Verification items for the finished model (mm, model axes). Face numbers are marked on the shaded views. Coordinates: 2 decimals unless noted, no trailing zeros. Order: outer loops, then holes, each group sorted by start corner. A loop starts at its lowest first (then second) coordinate and runs counter-clockwise, first axis right, second up. Notation, with made-up numbers: M 48,-15 L 103,-15 A18 cw 103,6 Z; hole C -22.75,57.25 d7. An arc over 180 degrees is marked long. Return JSON: item names as keys, results as strings.
```python
from build123d import *

# Parameters (mm, degrees)
SKETCH1_R                  = 63
SKETCH1_R_2                = 58
BOSS_EXTRUDE1_DEPTH        = 29.4
SKETCH2_R                  = 60.5
SKETCH2_R_2                = 58
CUT_EXTRUDE1_DEPTH         = 2
BOSS_EXTRUDE2_REACH        = 115.821
BOSS_EXTRUDE2_START_RADIUS = 63
BOSS_EXTRUDE2_END_RADIUS   = 63
SKETCH3_W                  = 60
SKETCH3_H                  = 29.4
SKETCH5_W                  = 29.4
SKETCH5_H                  = 24.463774017
CUT_EXTRUDE2_DEPTH         = 60
BOSS_EXTRUDE3_DEPTH        = 60
SKETCH7_W                  = 60
SKETCH7_H                  = 41.577878734
BOSS_EXTRUDE4_DEPTH        = 50
CUT_EXTRUDE3_REACH         = 173.878
SKETCH9_W                  = 60
SKETCH9_H                  = 50
BOSS_EXTRUDE5_DEPTH        = 26.14
SKETCH10_W                 = 60
SKETCH10_H                 = 26.14
BOSS_EXTRUDE6_DEPTH        = 30
SKETCH11_R                 = 58
CUT_EXTRUDE4_DEPTH         = 168.932327916
SKETCH14_W                 = 60
SKETCH14_H                 = 55.370879129
CUT_EXTRUDE5_DEPTH         = 14.7
CUT_EXTRUDE6_REACH         = 171.856
BOSS_EXTRUDE7_DEPTH        = 60
SKETCH17_R                 = 58
CUT_EXTRUDE7_DEPTH         = 155.195379415
SKETCH18_W                 = 60
SKETCH18_H                 = 15
CUT_EXTRUDE8_DEPTH         = 50
SKETCH19_R                 = 2
CUT_EXTRUDE9_DEPTH         = 15
SKETCH20_W                 = 60
SKETCH20_H                 = 20
CUT_EXTRUDE10_DEPTH        = 140.943357594


with BuildPart() as part:
    # Sketch1 → Boss-Extrude1 (new body)
    with BuildSketch(Plane.XY):
        Circle(SKETCH1_R)
        Circle(SKETCH1_R_2, mode=Mode.SUBTRACT)
    extrude(amount=BOSS_EXTRUDE1_DEPTH)

    # Sketch2 → Cut-Extrude1 (cut)
    with BuildSketch(Plane.XY.offset(29.4)):
        Circle(SKETCH2_R)
        Circle(SKETCH2_R_2, mode=Mode.SUBTRACT)
    extrude(amount=-CUT_EXTRUDE1_DEPTH, mode=Mode.SUBTRACT)

    # Boss-Extrude2: from a cylinder face, 115.821 long prism both ways, kept between that surface and its translate by the depth
    boss_extrude2_start = Plane(origin=(0, 0, 14.7), z_dir=(0, 0, -1)) * Cylinder(BOSS_EXTRUDE2_START_RADIUS, 358.642, mode=Mode.PRIVATE)
    boss_extrude2_end = Plane(origin=(0, 20, 14.7), z_dir=(0, 0, -1)) * Cylinder(BOSS_EXTRUDE2_END_RADIUS, 358.642, mode=Mode.PRIVATE)
    # Sketch3 → Boss-Extrude2 (add, from a surface)
    with BuildSketch(Plane(origin=(0, 0, 0), x_dir=(1, 0, 0), z_dir=(0, 1, 0)), mode=Mode.PRIVATE) as boss_extrude2_sk1:
        with Locations((0, -14.7)):
            Rectangle(SKETCH3_W, SKETCH3_H)
    boss_extrude2_tool1 = extrude(boss_extrude2_sk1.sketch, amount=BOSS_EXTRUDE2_REACH, both=True, mode=Mode.PRIVATE)
    add(((boss_extrude2_tool1 - boss_extrude2_start) & boss_extrude2_end).solids().sort_by_distance((0, 65.398556, 14.7))[0])

    # Sketch5 → Cut-Extrude2 (cut)
    with BuildSketch(Plane.ZY.offset(30)):
        with Locations((14.7, 87.630442947)):
            Rectangle(SKETCH5_W, SKETCH5_H)
    extrude(amount=-CUT_EXTRUDE2_DEPTH, mode=Mode.SUBTRACT)

    # Sketch6 → Boss-Extrude3 (add)
    with BuildSketch(Plane.ZY.offset(30)):
        Polygon((0, 75.398555938), (29.4, 104.798555938), (29.4, 75.398555938), align=None)
    extrude(amount=-BOSS_EXTRUDE3_DEPTH)

    # Sketch7 → Boss-Extrude4 (add)
    with BuildSketch(Plane(origin=(0, 37.699277969, -37.699277969), x_dir=(1, 0, 0), z_dir=(0, 0.7071067811865513, -0.7071067811865438))):
        with Locations((0, -74.103769562)):
            Rectangle(SKETCH7_W, SKETCH7_H)
    extrude(amount=BOSS_EXTRUDE4_DEPTH)

    # Sketch8 → Cut-Extrude3 (cut, up to next)
    with BuildSketch(Plane(origin=(30, 0, 0), x_dir=(0, 0, -1), z_dir=(1, 0, 0)), mode=Mode.PRIVATE) as cut_extrude3_sk1:
        Polygon((14.566399692, 131.542834364), (-29.4, 87.576434672), (-29.4, 104.798555938), (5.955339059, 140.153894997), align=None)
    cut_extrude3_tool1 = extrude(cut_extrude3_sk1.sketch, amount=-CUT_EXTRUDE3_REACH, mode=Mode.PRIVATE) & part.part
    add(cut_extrude3_tool1.solids().sort_by_distance((30, 115.784229, 9.491665))[0], mode=Mode.SUBTRACT)

    # Sketch9 → Boss-Extrude5 (add)
    with BuildSketch(Plane(origin=(0, 37.699277969, 37.699277969), x_dir=(1, 0, 0), z_dir=(0, -0.7071067811865438, -0.7071067811865512))):
        with Locations((0, -78.314830195)):
            Rectangle(SKETCH9_W, SKETCH9_H)
    extrude(amount=BOSS_EXTRUDE5_DEPTH)

    # Sketch10 → Boss-Extrude6 (add)
    with BuildSketch(Plane(origin=(0, 37.699277969, -37.699277969), x_dir=(1, 0, 0), z_dir=(0, -0.7071067811865511, 0.707106781186544))):
        with Locations((0, 40.244830195)):
            Rectangle(SKETCH10_W, SKETCH10_H)
    extrude(amount=BOSS_EXTRUDE6_DEPTH)

    # Sketch11 → Cut-Extrude4 (cut, through all)
    with BuildSketch(Plane.XY.offset(29.4)):
        with Locations(Location((0, 0, 0), (0, 0, 121.147389922))):
            Circle(SKETCH11_R)
    extrude(amount=-CUT_EXTRUDE4_DEPTH, mode=Mode.SUBTRACT)

    # Sketch14 → Cut-Extrude5 (cut)
    with BuildSketch(Plane.XY.offset(29.4)):
        with Locations((0, 115.261874237)):
            Rectangle(SKETCH14_W, SKETCH14_H)
        with BuildLine():
            ThreePointArc((30, 55.398555938), (0, 63), (-30, 55.398555938))
            Line((-30, 55.398555938), (-30, 87.576434672))
            Line((-30, 87.576434672), (30, 87.576434672))
            Line((30, 87.576434672), (30, 55.398555938))
        make_face()
    extrude(amount=-CUT_EXTRUDE5_DEPTH, mode=Mode.SUBTRACT)

    # Sketch15 → Cut-Extrude6 (cut, up to next)
    with BuildSketch(Plane(origin=(30, 0, 0), x_dir=(0, 0, -1), z_dir=(1, 0, 0)), mode=Mode.PRIVATE) as cut_extrude6_sk1:
        Polygon((32.625906884, 113.483327173), (-14.7, 66.157420289), (-14.7, 102.276434672), (14.566399692, 131.542834364), align=None)
    cut_extrude6_tool1 = extrude(cut_extrude6_sk1.sketch, amount=-CUT_EXTRUDE6_REACH, mode=Mode.PRIVATE) & part.part
    add(cut_extrude6_tool1.solids().sort_by_distance((30, 102.300453, -4.802927))[0], mode=Mode.SUBTRACT)

    # Sketch16 → Boss-Extrude7 (add)
    with BuildSketch(Plane(origin=(30, 0, 0), x_dir=(0, 0, -1), z_dir=(1, 0, 0))):
        Polygon((-14.7, 66.157420289), (-25.458864351, 55.398555938), (-14.7, 55.398555938), align=None)
    extrude(amount=-BOSS_EXTRUDE7_DEPTH)

    # Sketch17 → Cut-Extrude7 (cut, through all)
    with BuildSketch(Plane.XY.offset(29.4)):
        with Locations(Location((0, 0, 0), (0, 0, 121.147389922))):
            Circle(SKETCH17_R)
    extrude(amount=-CUT_EXTRUDE7_DEPTH, mode=Mode.SUBTRACT)

    # Sketch18 → Cut-Extrude8 (cut)
    with BuildSketch(Plane(origin=(0, 73.054617028, -73.054617028), x_dir=(1, 0, 0), z_dir=(0, 0.7071067811865512, -0.7071067811865438))):
        with Locations((0, -49.674830195)):
            Rectangle(SKETCH18_W, SKETCH18_H)
    extrude(amount=-CUT_EXTRUDE8_DEPTH, mode=Mode.SUBTRACT)

    # Sketch19 → Cut-Extrude9 (cut)
    with BuildSketch(Plane(origin=(0, 19.215506709, 19.215506709), x_dir=(1, 0, 0), z_dir=(0, -0.7071067811865438, -0.7071067811865512))):
        with Locations(Location((15, -67.788834976, 0), (0, 0, 270))):
            Circle(SKETCH19_R)
        with Locations(Location((-15, -67.788834976, 0), (0, 0, 270))):
            Circle(SKETCH19_R)
    extrude(amount=-CUT_EXTRUDE9_DEPTH, mode=Mode.SUBTRACT)

    # Sketch20 → Cut-Extrude10 (cut, through all)
    with BuildSketch(Plane(origin=(0, 29.822108427, 29.822108427), x_dir=(1, 0, 0), z_dir=(0, 0.7071067811865438, 0.7071067811865513))):
        with Locations((0, 93.314830195)):
            Rectangle(SKETCH20_W, SKETCH20_H)
    extrude(amount=-CUT_EXTRUDE10_DEPTH, mode=Mode.SUBTRACT)


solid = part.part
```
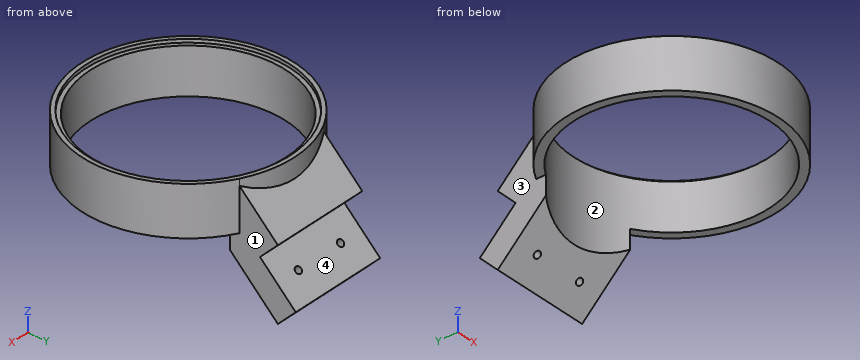
Q1. Cross-section at A-A, the plane y = 0. Record the boundary of the cut face in (x, z).
Values:
{"outline": "M -63,0 L -58,0 L -58,27.4 L -60.5,27.4 L -60.5,29.4 L -63,29.4 Z; M 58,0 L 63,0 L 63,29.4 L 60.5,29.4 L 60.5,27.4 L 58,27.4 Z"}
Q2. Cross-section at B-B, the plane x = 0. Record the boundary of the cut face in (y, z).
Values:
{"outline": "M -63,0 L -58,0 L -58,27.4 L -60.5,27.4 L -60.5,29.4 L -63,29.4 Z; M 58,-19.57 L 78.13,-39.7 L 88.73,-29.09 L 67.52,-7.88 L 78.13,2.73 L 63,17.86 L 63,29.4 L 60.5,29.4 L 60.5,27.4 L 58,27.4 Z"}
Q3. Go/stop test with flat-tipped pins: pin 1 (19.5 mm diameter, centred on y = 64.5, z = 3.5, fed in from -X); pin 2 (5 mm diameter, centred on y = 65, z = -17, fed in from +X); pin 3 (12 mm diameter, centred on x = -9.5, z = -29.5, fed in from -Y). Record where each tip stops, or that it passes through.
Values:
{"pin 1": "x = -31.17", "pin 2": "x = 30", "pin 3": "y = 61.93"}
Q4. Draft check along X on the marked faces 1, 2, 3 and 4. Enter one of: pulls with the +X half, pulls with the -X half, needs draft (parallel to the pull), parting line crosses it, or undercut.
Values:
{"face 1": "pulls with the +X half", "face 2": "undercut", "face 3": "pulls with the -X half", "face 4": "needs draft"}
Q5. Material ranges on line 1 along X through (y, z) = (0, 8); line 2 along Y through (x, z) = (0, 28.35); line 3 along Z through (x, y) = (-16, 70), recorded low to high.
Values:
{"line 1": "-63 to -58, 58 to 63", "line 2": "-63 to -60.5, 60.5 to 63", "line 3": "-31.57 to -28.32, -23.42 to -10.36, -5.4 to 10.86"}
Q6. Cross-section at D-D, the plane z = -15. Record the boundary of the cut face in (x, y).
Values:
{"outline": "M -30,53.43 L -22.56,53.43 A58 cw 22.56,53.43 L 30,53.43 L 30,74.64 L -30,74.64 Z"}
Q7. Cross-section at C-C, the plane y = -46.5. Record the boundary of the cut face in (x, z).
Values:
{"outline": "M -42.51,0 L -34.67,0 L -34.67,27.4 L -38.7,27.4 L -38.7,29.4 L -42.51,29.4 Z; M 34.67,0 L 42.51,0 L 42.51,29.4 L 38.7,29.4 L 38.7,27.4 L 34.67,27.4 Z"}
